Could you check a few things on this model? Use its own coordinates, in mm. A direction names the side the tool comes from. Round coordinates to 2 decimals unless told otherwise and drop trailing zeros. Write each loop counter-clockwise with the first axis right and the second up, starting at its lowest first coordinate (ties: lowest second). Pieces come first, ordered by that corner, then holes. Notation, with made-up numbers: (-20, 33) -> (7, 33) arc R25 cw to (7, 56) -> close; hole circle Ø8 at (28.5, 22.25). An arc over 180 degrees is marked (long way). Answer in a Markdown table with one row per item.
from build123d import *

# Parameters (mm, degrees)
SKETCH1_W           = 88.6
SKETCH1_H           = 7.2
SKETCH1_W_2         = 68
SKETCH1_H_2         = 6
SKETCH1_R           = 1.375
BOSS_EXTRUDE1_DEPTH = 1.6


with BuildPart() as part:
    # Sketch1 → Boss-Extrude1 (new body)
    with BuildSketch(Plane(origin=(0, 0, 0), x_dir=(1, 0, 0), z_dir=(0, 1, 0))):
        with Locations((9.305038693, -28.915060123)):
            Rectangle(SKETCH1_W, SKETCH1_H)
        with Locations((9.305038693, -22.315060123)):
            Rectangle(SKETCH1_W_2, SKETCH1_H_2)
        with Locations((-22.694961307, -21.362291366)):
            Circle(SKETCH1_R, mode=Mode.SUBTRACT)
        with Locations((41.305038693, -21.362291366)):
            Circle(SKETCH1_R, mode=Mode.SUBTRACT)
    extrude(amount=BOSS_EXTRUDE1_DEPTH)


solid = part.part
1) For faces 5 (the face through (48, 1, 25.315)), 6 (the face through (9, 1, 32.515)), 7 (the face through (-30, 1, 25.315)), which set-ups out of +Z, -Z, +X, -X, +Y, -Y let a thin tool reach every point of the face, with its end or its side?
Findings:
| item | result |
|---|---|
| face 5 | -Z, +X, +Y, -Y |
| face 6 | +Z, +X, -X, +Y, -Y |
| face 7 | -Z, -X, +Y, -Y |
2) Please list where these lines run through material, in increasing order: line 1 (X direction, y = 1.1, z = 24.75); line 2 (X direction, y = 1.45, z = 22); line 3 (X direction, y = 1.2, z = 22.25) (3 decimals).
Findings:
| item | result |
|---|---|
| line 1 | x = -24.69 to 43.31 |
| line 2 | x = -24.69 to -23.91, -21.48 to 40.09, 42.52 to 43.31 |
| line 3 | x = -24.695 to -23.745, -21.645 to 40.255, 42.355 to 43.305 |
3) Imagine slicing it at B-B, the plane z = 24.25. Please give me the cut outline in (x, y).
Findings:
| item | result |
|---|---|
| outline | (-24.69, 0) -> (43.31, 0) -> (43.31, 1.6) -> (-24.69, 1.6) -> close |
4) For pin 1 (1.5 mm diameter, centred on x = -3.5, z = 22.5, fed in from -Y), with a flat end and sliding along its axis, tell me the tip position at first contact or that it passes through.
Findings:
| item | result |
|---|---|
| pin 1 | stops at y = 0 |
5) Thinking about a two-plate mould opening in X: for faces 1 (the face through (9, 1, 19.315)), 2 (the face through (39.93, 0.79, 21.3)), 3 (the face through (-21.96, 0.79, 20.2)), 4 (the face through (53.605, 1, 29)), which applies, +X half, -X half, draft (parallel to the pull), parting line (faces both ways), or undercut?
Findings:
| item | result |
|---|---|
| face 1 | draft |
| face 2 | undercut |
| face 3 | undercut |
| face 4 | +X half |
6) Imagine slicing it at A-A, the plane y = 0.3. Please give me the cut outline in (x, z) (3 decimals), plus the area to 3 significant figures.
Findings:
| item | result |
|---|---|
| outline | (-34.995, 25.315) -> (-24.695, 25.315) -> (-24.695, 19.315) -> (43.305, 19.315) -> (43.305, 25.315) -> (53.605, 25.315) -> (53.605, 32.515) -> (-34.995, 32.515) -> close; hole circle Ø2.75 at (-22.695, 21.362); hole circle Ø2.75 at (41.305, 21.362) |
| area | 1,030 mm^2 |
